Geometry: final body of the model. Coordinates: model frame, mm. A direction names the side the tool comes from. Coordinates: 2 decimals unless noted, no trailing zeros. Order: outer loops, then holes, each group sorted by start corner. A loop starts at its lowest first (then second) coordinate and runs counter-clockwise, first axis right, second up. Notation, with made-up numbers: M 60,10.5 L 92,10.5 A19 cw 92,47.5 Z; hole C 31.25,30 d10. An arc over 180 degrees is marked long. Use CSV: the item, a comma, the result in double quotes. Start each with the question number.
1. Pull-direction query (Z, two-part tool) for faces 1 (the flat face through (189, 5, 18)), 2 (the flat face through (239, 5, 54)); classes: pulls with the +Z half, pulls with the -Z half, needs draft (parallel to the pull), parting line crosses it, or undercut.
2. Set-up query: faces 3 (the flat face through (224, 5, -92)), 4 (the flat face through (-3, 0, 125)), 5 (the flat face through (-145, 5, 149)). Return all of +Z, -Z, +X, -X, +Y, -Y with unobstructed straight access to the full face (end or side cutting, diameter ignored); none if empty.
3. Section query B-B on x = 20. Return the cut outline in (y, z), and give its area (3 significant figures).
4. Material intervals for line 1 (X direction, y = 5, z = -5); line 2 (Z direction, x = -80.5, y = 6); line 3 (Z direction, x = 126.5, y = 2.75), sorted ascending.
5. Section query C-C on z = 91.5. Return the cut outline in (x, y).
6. Section query D-D on x = 94. Return the cut outline in (y, z), and give its area (3 significant figures).
7. Section query A-A on z = -100. Return the cut outline in (x, y), and give its area (3 significant figures).
8. First-contact query: P1, Ø10, axis at x = 151.5, z = 3.5, coming from the -Y side. Flat tip, straight axial feed; report the tip coordinate or a pass-through.
from build123d import *

# Parameters (mm, degrees)
SKETCH1_W           = 478
SKETCH1_H           = 328
BOSS_EXTRUDE1_DEPTH = 10
CUT_EXTRUDE1_REACH  = 302.396
SKETCH2_W           = 20
SKETCH2_H           = 20
CUT_EXTRUDE2_REACH  = 302.396
SKETCH3_W           = 290
SKETCH3_H           = 10
SKETCH3_W_2         = 10
SKETCH3_H_2         = 39
SKETCH3_W_3         = 39
SKETCH3_W_4         = 70
SKETCH3_H_3         = 25
SKETCH3_H_4         = 180
SKETCH3_W_5         = 15
SKETCH3_H_5         = 30


with BuildPart() as part:
    # Sketch1 → Boss-Extrude1 (new body)
    with BuildSketch(Plane(origin=(0, 0, 0), x_dir=(1, 0, 0), z_dir=(0, 1, 0))):
        with Locations((0, -17.705479187)):
            Rectangle(SKETCH1_W, SKETCH1_H)
    extrude(amount=BOSS_EXTRUDE1_DEPTH)

    # Sketch2 → Cut-Extrude1 (cut, up to next)
    with BuildSketch(Plane(origin=(0, 10, 0), x_dir=(1, 0, 0), z_dir=(0, 1, 0)), mode=Mode.PRIVATE) as cut_extrude1_sk1:
        with Locations((-225, 132.294520813)):
            Rectangle(SKETCH2_W, SKETCH2_H)
    cut_extrude1_tool1 = extrude(cut_extrude1_sk1.sketch, amount=-CUT_EXTRUDE1_REACH, mode=Mode.PRIVATE) & part.part
    # Sketch2 → Cut-Extrude1 (cut, up to next)
    with BuildSketch(Plane(origin=(0, 10, 0), x_dir=(1, 0, 0), z_dir=(0, 1, 0)), mode=Mode.PRIVATE) as cut_extrude1_sk2:
        with Locations((-225, -167.705479187)):
            Rectangle(SKETCH2_W, SKETCH2_H)
    cut_extrude1_tool2 = extrude(cut_extrude1_sk2.sketch, amount=-CUT_EXTRUDE1_REACH, mode=Mode.PRIVATE) & part.part
    # Sketch2 → Cut-Extrude1 (cut, up to next)
    with BuildSketch(Plane(origin=(0, 10, 0), x_dir=(1, 0, 0), z_dir=(0, 1, 0)), mode=Mode.PRIVATE) as cut_extrude1_sk3:
        with Locations((225, 132.294520813)):
            Rectangle(SKETCH2_W, SKETCH2_H)
    cut_extrude1_tool3 = extrude(cut_extrude1_sk3.sketch, amount=-CUT_EXTRUDE1_REACH, mode=Mode.PRIVATE) & part.part
    # Sketch2 → Cut-Extrude1 (cut, up to next)
    with BuildSketch(Plane(origin=(0, 10, 0), x_dir=(1, 0, 0), z_dir=(0, 1, 0)), mode=Mode.PRIVATE) as cut_extrude1_sk4:
        with Locations((225, -167.705479187)):
            Rectangle(SKETCH2_W, SKETCH2_H)
    cut_extrude1_tool4 = extrude(cut_extrude1_sk4.sketch, amount=-CUT_EXTRUDE1_REACH, mode=Mode.PRIVATE) & part.part
    add(cut_extrude1_tool1.solids().sort_by_distance((-225, 10, -132.294521))[0], mode=Mode.SUBTRACT)
    add(cut_extrude1_tool2.solids().sort_by_distance((-225, 10, 167.705479))[0], mode=Mode.SUBTRACT)
    add(cut_extrude1_tool3.solids().sort_by_distance((225, 10, -132.294521))[0], mode=Mode.SUBTRACT)
    add(cut_extrude1_tool4.solids().sort_by_distance((225, 10, 167.705479))[0], mode=Mode.SUBTRACT)

    # Sketch3 → Cut-Extrude2 (cut, up to next)
    with BuildSketch(Plane(origin=(0, 10, 0), x_dir=(1, 0, 0), z_dir=(0, 1, 0)), mode=Mode.PRIVATE) as cut_extrude2_sk1:
        with Locations((0, 131.294520813)):
            Rectangle(SKETCH3_W, SKETCH3_H)
    cut_extrude2_tool1 = extrude(cut_extrude2_sk1.sketch, amount=-CUT_EXTRUDE2_REACH, mode=Mode.PRIVATE) & part.part
    # Sketch3 → Cut-Extrude2 (cut, up to next)
    with BuildSketch(Plane(origin=(0, 10, 0), x_dir=(1, 0, 0), z_dir=(0, 1, 0)), mode=Mode.PRIVATE) as cut_extrude2_sk2:
        with Locations((-200, 91.794520813)):
            Rectangle(SKETCH3_W_2, SKETCH3_H_2)
    cut_extrude2_tool2 = extrude(cut_extrude2_sk2.sketch, amount=-CUT_EXTRUDE2_REACH, mode=Mode.PRIVATE) & part.part
    # Sketch3 → Cut-Extrude2 (cut, up to next)
    with BuildSketch(Plane(origin=(0, 10, 0), x_dir=(1, 0, 0), z_dir=(0, 1, 0)), mode=Mode.PRIVATE) as cut_extrude2_sk3:
        with Locations((200, 91.794520813)):
            Rectangle(SKETCH3_W_2, SKETCH3_H_2)
    cut_extrude2_tool3 = extrude(cut_extrude2_sk3.sketch, amount=-CUT_EXTRUDE2_REACH, mode=Mode.PRIVATE) & part.part
    # Sketch3 → Cut-Extrude2 (cut, up to next)
    with BuildSketch(Plane(origin=(0, 10, 0), x_dir=(1, 0, 0), z_dir=(0, 1, 0)), mode=Mode.PRIVATE) as cut_extrude2_sk4:
        with Locations((200, -127.205479187)):
            Rectangle(SKETCH3_W_2, SKETCH3_H_2)
    cut_extrude2_tool4 = extrude(cut_extrude2_sk4.sketch, amount=-CUT_EXTRUDE2_REACH, mode=Mode.PRIVATE) & part.part
    # Sketch3 → Cut-Extrude2 (cut, up to next)
    with BuildSketch(Plane(origin=(0, 10, 0), x_dir=(1, 0, 0), z_dir=(0, 1, 0)), mode=Mode.PRIVATE) as cut_extrude2_sk5:
        with Locations((-200, -127.205479187)):
            Rectangle(SKETCH3_W_2, SKETCH3_H_2)
    cut_extrude2_tool5 = extrude(cut_extrude2_sk5.sketch, amount=-CUT_EXTRUDE2_REACH, mode=Mode.PRIVATE) & part.part
    # Sketch3 → Cut-Extrude2 (cut, up to next)
    with BuildSketch(Plane(origin=(0, 10, 0), x_dir=(1, 0, 0), z_dir=(0, 1, 0)), mode=Mode.PRIVATE) as cut_extrude2_sk6:
        with Locations((-125.5, -148.705479187)):
            Rectangle(SKETCH3_W_3, SKETCH3_H)
    cut_extrude2_tool6 = extrude(cut_extrude2_sk6.sketch, amount=-CUT_EXTRUDE2_REACH, mode=Mode.PRIVATE) & part.part
    # Sketch3 → Cut-Extrude2 (cut, up to next)
    with BuildSketch(Plane(origin=(0, 10, 0), x_dir=(1, 0, 0), z_dir=(0, 1, 0)), mode=Mode.PRIVATE) as cut_extrude2_sk7:
        with Locations((125.5, -148.705479187)):
            Rectangle(SKETCH3_W_3, SKETCH3_H)
    cut_extrude2_tool7 = extrude(cut_extrude2_sk7.sketch, amount=-CUT_EXTRUDE2_REACH, mode=Mode.PRIVATE) & part.part
    # Sketch3 → Cut-Extrude2 (cut, up to next)
    with BuildSketch(Plane(origin=(0, 10, 0), x_dir=(1, 0, 0), z_dir=(0, 1, 0)), mode=Mode.PRIVATE) as cut_extrude2_sk8:
        with Locations((0, -156.205479187)):
            Rectangle(SKETCH3_W_4, SKETCH3_H_3)
    cut_extrude2_tool8 = extrude(cut_extrude2_sk8.sketch, amount=-CUT_EXTRUDE2_REACH, mode=Mode.PRIVATE) & part.part
    # Sketch3 → Cut-Extrude2 (cut, up to next)
    with BuildSketch(Plane(origin=(0, 10, 0), x_dir=(1, 0, 0), z_dir=(0, 1, 0)), mode=Mode.PRIVATE) as cut_extrude2_sk9:
        with BuildLine():
            Line((-204, -60.205479187), (-194, -60.205479187))
            ThreePointArc((-194, -60.205479187), (-190.464466094, -58.741013093), (-189, -55.205479187))
            Line((-189, -55.205479187), (-189, 19.794520813))
            ThreePointArc((-189, 19.794520813), (-190.464466094, 23.330054719), (-194, 24.794520813))
            Line((-194, 24.794520813), (-204, 24.794520813))
            ThreePointArc((-204, 24.794520813), (-207.535533906, 23.330054719), (-209, 19.794520813))
            Line((-209, 19.794520813), (-209, -55.205479187))
            ThreePointArc((-209, -55.205479187), (-207.535533906, -58.741013093), (-204, -60.205479187))
        make_face()
    cut_extrude2_tool9 = extrude(cut_extrude2_sk9.sketch, amount=-CUT_EXTRUDE2_REACH, mode=Mode.PRIVATE) & part.part
    # Sketch3 → Cut-Extrude2 (cut, up to next)
    with BuildSketch(Plane(origin=(0, 10, 0), x_dir=(1, 0, 0), z_dir=(0, 1, 0)), mode=Mode.PRIVATE) as cut_extrude2_sk10:
        with BuildLine():
            Line((189, -55.205479187), (189, 19.794520813))
            ThreePointArc((189, 19.794520813), (190.464466094, 23.330054719), (194, 24.794520813))
            Line((194, 24.794520813), (204, 24.794520813))
            ThreePointArc((204, 24.794520813), (207.535533906, 23.330054719), (209, 19.794520813))
            Line((209, 19.794520813), (209, -55.205479187))
            ThreePointArc((209, -55.205479187), (207.535533906, -58.741013093), (204, -60.205479187))
            Line((204, -60.205479187), (194, -60.205479187))
            ThreePointArc((194, -60.205479187), (190.464466094, -58.741013093), (189, -55.205479187))
        make_face()
    cut_extrude2_tool10 = extrude(cut_extrude2_sk10.sketch, amount=-CUT_EXTRUDE2_REACH, mode=Mode.PRIVATE) & part.part
    # Sketch3 → Cut-Extrude2 (cut, up to next)
    with BuildSketch(Plane(origin=(0, 10, 0), x_dir=(1, 0, 0), z_dir=(0, 1, 0)), mode=Mode.PRIVATE) as cut_extrude2_sk11:
        with Locations((0, -17.705479187)):
            Rectangle(SKETCH3_W, SKETCH3_H_4)
    cut_extrude2_tool11 = extrude(cut_extrude2_sk11.sketch, amount=-CUT_EXTRUDE2_REACH, mode=Mode.PRIVATE) & part.part
    # Sketch3 → Cut-Extrude2 (cut, up to next)
    with BuildSketch(Plane(origin=(0, 10, 0), x_dir=(1, 0, 0), z_dir=(0, 1, 0)), mode=Mode.PRIVATE) as cut_extrude2_sk12:
        with Locations((-231.5, 92.294520813)):
            Rectangle(SKETCH3_W_5, SKETCH3_H_5)
    cut_extrude2_tool12 = extrude(cut_extrude2_sk12.sketch, amount=-CUT_EXTRUDE2_REACH, mode=Mode.PRIVATE) & part.part
    # Sketch3 → Cut-Extrude2 (cut, up to next)
    with BuildSketch(Plane(origin=(0, 10, 0), x_dir=(1, 0, 0), z_dir=(0, 1, 0)), mode=Mode.PRIVATE) as cut_extrude2_sk13:
        with Locations((231.5, 92.294520813)):
            Rectangle(SKETCH3_W_5, SKETCH3_H_5)
    cut_extrude2_tool13 = extrude(cut_extrude2_sk13.sketch, amount=-CUT_EXTRUDE2_REACH, mode=Mode.PRIVATE) & part.part
    add(cut_extrude2_tool1.solids().sort_by_distance((0, 10, -131.294521))[0], mode=Mode.SUBTRACT)
    add(cut_extrude2_tool2.solids().sort_by_distance((-200, 10, -91.794521))[0], mode=Mode.SUBTRACT)
    add(cut_extrude2_tool3.solids().sort_by_distance((200, 10, -91.794521))[0], mode=Mode.SUBTRACT)
    add(cut_extrude2_tool4.solids().sort_by_distance((200, 10, 127.205479))[0], mode=Mode.SUBTRACT)
    add(cut_extrude2_tool5.solids().sort_by_distance((-200, 10, 127.205479))[0], mode=Mode.SUBTRACT)
    add(cut_extrude2_tool6.solids().sort_by_distance((-125.5, 10, 148.705479))[0], mode=Mode.SUBTRACT)
    add(cut_extrude2_tool7.solids().sort_by_distance((125.5, 10, 148.705479))[0], mode=Mode.SUBTRACT)
    add(cut_extrude2_tool8.solids().sort_by_distance((0, 10, 156.205479))[0], mode=Mode.SUBTRACT)
    add(cut_extrude2_tool9.solids().sort_by_distance((-199, 10, 17.705479))[0], mode=Mode.SUBTRACT)
    add(cut_extrude2_tool10.solids().sort_by_distance((199, 10, 17.705479))[0], mode=Mode.SUBTRACT)
    add(cut_extrude2_tool11.solids().sort_by_distance((0, 10, 17.705479))[0], mode=Mode.SUBTRACT)
    add(cut_extrude2_tool12.solids().sort_by_distance((-231.5, 10, -92.294521))[0], mode=Mode.SUBTRACT)
    add(cut_extrude2_tool13.solids().sort_by_distance((231.5, 10, -92.294521))[0], mode=Mode.SUBTRACT)


solid = part.part
Results list:
1,face 1,"undercut"
1,face 2,"needs draft"
2,face 3,"+X, +Y, -Y"
2,face 4,"+Z, -Z, +X, -X, -Y"
2,face 5,"+Y, -Y"
3,outline,"M 0,-146.29 L 10,-146.29 L 10,-136.29 L 0,-136.29 Z; M 0,-126.29 L 10,-126.29 L 10,-72.29 L 0,-72.29 Z; M 0,107.71 L 10,107.71 L 10,143.71 L 0,143.71 Z; M 0,168.71 L 10,168.71 L 10,181.71 L 0,181.71 Z"
3,area,"1,130 mm²"
4,line 1,"x = -239 to -209, -189 to -145, 145 to 189, 209 to 239"
4,line 2,"z = -146.29 to -136.29, -126.29 to -72.29, 107.71 to 181.71"
4,line 3,"z = -146.29 to -136.29, -126.29 to -72.29, 107.71 to 143.71, 153.71 to 181.71"
5,outline,"M -239,0 L -145,0 L -145,10 L -239,10 Z; M 145,0 L 239,0 L 239,10 L 145,10 Z"
6,outline,"M 0,-146.29 L 10,-146.29 L 10,-136.29 L 0,-136.29 Z; M 0,-126.29 L 10,-126.29 L 10,-72.29 L 0,-72.29 Z; M 0,107.71 L 10,107.71 L 10,181.71 L 0,181.71 Z"
6,area,"1,380 mm²"
7,outline,"M -224,0 L -205,0 L -205,10 L -224,10 Z; M -195,0 L 195,0 L 195,10 L -195,10 Z; M 205,0 L 224,0 L 224,10 L 205,10 Z"
7,area,"4,280 mm²"
8,P1,"stops at y = 0"
